Design review of the part built by this model. Coordinates are the model's own, in mm. Face numbers are marked on the shaded views. Round coordinates to 2 decimals unless told otherwise and drop trailing zeros. Order: outer loops, then holes, each group sorted by start corner. A loop starts at its lowest first (then second) coordinate and runs counter-clockwise, first axis right, second up.
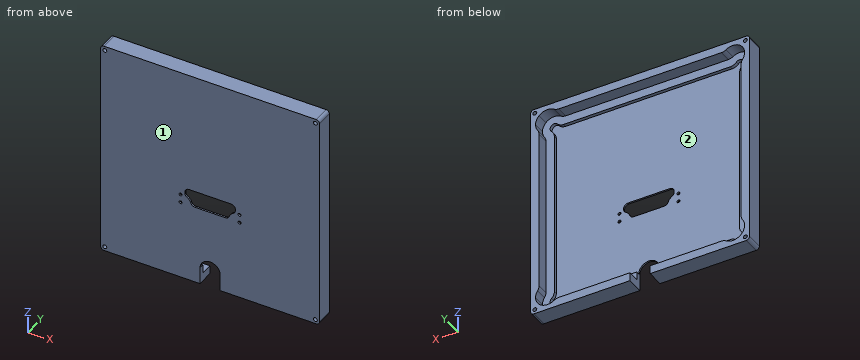
from build123d import *

# Parameters (mm, degrees)
SKETCH2_W           = 165.1
SKETCH2_H           = 165.1
BOSS_EXTRUDE1_DEPTH = 12.7
SKETCH3_W           = 152.4
SKETCH3_H           = 152.4
CUT_EXTRUDE1_DEPTH  = 8.9027
SKETCH4_W           = 139.7
SKETCH4_H           = 139.7
CUT_EXTRUDE2_DEPTH  = 2.54
SKETCH5_R           = 1.1303
CUT_EXTRUDE4_DEPTH  = 234.766882563
SKETCH6_R           = 1.4732
CUT_EXTRUDE5_DEPTH  = 234.831798522
FILLET2_R           = 2.54
CUT_EXTRUDE6_DEPTH  = 234.831798522
CUT_EXTRUDE11_DEPTH = 8.9027
SKETCH9_R           = 3.175
CUT_EXTRUDE12_DEPTH = 2.54
FILLET3_R           = 6.35
FILLET4_R           = 6.35
FILLET5_START       = -1
FILLET5_DEPTH       = 3
FILLET6_R           = 3.175


with BuildPart() as part:
    # Sketch2 → Boss-Extrude1 (new body)
    with BuildSketch(Plane(origin=(0, 0, 0), x_dir=(1, 0, 0), z_dir=(0, 1, 0))):
        with Locations((82.55, 82.55)):
            Rectangle(SKETCH2_W, SKETCH2_H)
    extrude(amount=BOSS_EXTRUDE1_DEPTH)

    # Sketch3 → Cut-Extrude1 (cut)
    with BuildSketch(Plane(origin=(0, 12.7, 0), x_dir=(1, 0, 0), z_dir=(0, 1, 0))):
        with Locations((82.55, 82.55)):
            Rectangle(SKETCH3_W, SKETCH3_H)
    extrude(amount=-CUT_EXTRUDE1_DEPTH, mode=Mode.SUBTRACT)

    # Sketch4 → Cut-Extrude2 (cut)
    with BuildSketch(Plane(origin=(0, 3.7973, 0), x_dir=(1, 0, 0), z_dir=(0, 1, 0))):
        with Locations((82.55, 82.55)):
            Rectangle(SKETCH4_W, SKETCH4_H)
    extrude(amount=-CUT_EXTRUDE2_DEPTH, mode=Mode.SUBTRACT)

    # Sketch5 → Cut-Extrude4 (cut, through all)
    with BuildSketch(Plane(origin=(0, 1.2573, 0), x_dir=(1, 0, 0), z_dir=(0, 1, 0))):
        with BuildLine():
            Line((93.98, 104.775), (71.12, 104.775))
            ThreePointArc((71.12, 104.775), (67.945, 101.6), (71.12, 98.425))
            Line((71.12, 98.425), (93.98, 98.425))
            ThreePointArc((93.98, 98.425), (97.155, 101.6), (93.98, 104.775))
        make_face()
        with Locations(Location((60.325, 98.425, 0), (0, 0, 270))):
            Circle(SKETCH5_R)
        with Locations(Location((104.775, 98.425, 0), (0, 0, 270))):
            Circle(SKETCH5_R)
        Polygon((101.6, 98.425), (93.98, 98.425), (71.12, 98.425), (63.5, 98.425), (63.5, 92.075), (101.6, 92.075), align=None)
        with Locations(Location((60.325, 104.775, 0), (0, 0, 270))):
            Circle(SKETCH5_R)
        with Locations(Location((104.775, 104.775, 0), (0, 0, 90))):
            Circle(SKETCH5_R)
    extrude(amount=-CUT_EXTRUDE4_DEPTH, mode=Mode.SUBTRACT)

    # Sketch6 → Cut-Extrude5 (cut, through all)
    with BuildSketch(Plane(origin=(0, 12.7, 0), x_dir=(1, 0, 0), z_dir=(0, 1, 0))):
        with Locations(Location((3.175, 161.925, 0), (0, 0, 270))):
            Circle(SKETCH6_R)
        with Locations(Location((161.925, 161.925, 0), (0, 0, 90))):
            Circle(SKETCH6_R)
        with Locations(Location((161.925, 3.175, 0), (0, 0, 270))):
            Circle(SKETCH6_R)
        with Locations(Location((3.175, 3.175, 0), (0, 0, 90))):
            Circle(SKETCH6_R)
    extrude(amount=-CUT_EXTRUDE5_DEPTH, mode=Mode.SUBTRACT)

    # Fillet2
    fillet2_edges = [part.edges().sort_by_distance(p)[0] for p in [
        (0, 6.35, -165.1),
        (165.1, 6.35, -165.1),
        (165.1, 6.35, 0),
        (0, 6.35, 0),
    ]]
    fillet(fillet2_edges, radius=FILLET2_R)

    # Sketch7 → Cut-Extrude6 (cut, through all)
    with BuildSketch(Plane(origin=(0, 12.7, 0), x_dir=(1, 0, 0), z_dir=(0, 1, 0))):
        with BuildLine():
            Line((74.93, 152.4), (74.93, 165.1))
            ThreePointArc((74.93, 165.1), (82.55, 172.72), (90.17, 165.1))
            Line((90.17, 165.1), (90.17, 152.4))
            ThreePointArc((90.17, 152.4), (82.55, 144.78), (74.93, 152.4))
        make_face()
    extrude(amount=-CUT_EXTRUDE6_DEPTH, mode=Mode.SUBTRACT)

    # Sketch8 → Cut-Extrude11 (cut)
    with BuildSketch(Plane(origin=(0, 12.7, 0), x_dir=(1, 0, 0), z_dir=(0, 1, 0))):
        with BuildLine():
            Line((6.35, 152.4), (6.35, 158.75))
            ThreePointArc((6.35, 158.75), (3.719743879, 152.4), (6.35, 146.05))
            Line((6.35, 146.05), (6.35, 152.4))
        make_face()
        with BuildLine():
            ThreePointArc((19.05, 158.75), (12.7, 161.380256121), (6.35, 158.75))
            Line((6.35, 158.75), (12.7, 158.75))
            Line((12.7, 158.75), (19.05, 158.75))
        make_face()
        with BuildLine():
            Line((6.35, 12.7), (6.35, 19.05))
            ThreePointArc((6.35, 19.05), (3.719743879, 12.7), (6.35, 6.35))
            Line((6.35, 6.35), (6.35, 12.7))
        make_face()
        with BuildLine():
            Line((12.7, 6.35), (6.35, 6.35))
            ThreePointArc((6.35, 6.35), (12.7, 3.719743879), (19.05, 6.35))
            Line((19.05, 6.35), (12.7, 6.35))
        make_face()
        with BuildLine():
            Line((152.4, 6.35), (146.05, 6.35))
            ThreePointArc((146.05, 6.35), (152.4, 3.719743879), (158.75, 6.35))
            Line((158.75, 6.35), (152.4, 6.35))
        make_face()
        with BuildLine():
            ThreePointArc((161.380256121, 12.7), (160.696674827, 16.136595236), (158.75, 19.05))
            Line((158.75, 19.05), (158.75, 12.7))
            Line((158.75, 12.7), (158.75, 6.35))
            ThreePointArc((158.75, 6.35), (160.696674827, 9.263404764), (161.380256121, 12.7))
        make_face()
        with BuildLine():
            Line((158.75, 152.4), (158.75, 146.05))
            ThreePointArc((158.75, 146.05), (160.696674827, 148.963404764), (161.380256121, 152.4))
            ThreePointArc((161.380256121, 152.4), (160.696674827, 155.836595236), (158.75, 158.75))
            Line((158.75, 158.75), (158.75, 152.4))
        make_face()
        with BuildLine():
            ThreePointArc((158.75, 158.75), (152.4, 161.380256121), (146.05, 158.75))
            Line((146.05, 158.75), (152.4, 158.75))
            Line((152.4, 158.75), (158.75, 158.75))
        make_face()
    extrude(amount=-CUT_EXTRUDE11_DEPTH, mode=Mode.SUBTRACT)

    # Sketch9 → Cut-Extrude12 (cut)
    with BuildSketch(Plane(origin=(0, 3.7973, 0), x_dir=(1, 0, 0), z_dir=(0, 1, 0))):
        with Locations((12.7, 152.4)):
            Circle(SKETCH9_R)
        with Locations((152.4, 152.4)):
            Circle(SKETCH9_R)
        with Locations((152.4, 12.7)):
            Circle(SKETCH9_R)
        with Locations((12.7, 12.7)):
            Circle(SKETCH9_R)
    extrude(amount=-CUT_EXTRUDE12_DEPTH, mode=Mode.SUBTRACT)

    # Fillet3
    fillet3_edges = [part.edges().sort_by_distance(p)[0] for p in [
        (149.225, 2.5273, -12.7),
        (15.875, 2.5273, -12.7),
        (152.4, 2.5273, -149.225),
        (12.7, 2.5273, -149.225),
        (12.7, 2.5273, -15.875),
        (152.4, 2.5273, -15.875),
        (149.225, 2.5273, -152.4),
        (15.875, 2.5273, -152.4),
    ]]
    fillet(fillet3_edges, radius=FILLET3_R)

    # Fillet4
    fillet4_edges = [part.edges().sort_by_distance(p)[0] for p in [
        (146.05, 8.24865, -158.75),
        (146.05, 8.24865, -6.35),
        (19.05, 8.24865, -6.35),
        (6.35, 8.24865, -146.05),
        (19.05, 8.24865, -158.75),
        (6.35, 8.24865, -19.05),
        (158.75, 8.24865, -19.05),
        (158.75, 8.24865, -146.05),
    ]]
    fillet(fillet4_edges, radius=FILLET4_R)

    # Fillet5: read off the stored shape, not the designer's step
    # Fillet5 outline → Fillet5 (cut)
    with BuildSketch(Plane(origin=(0, 0, 0), x_dir=(1, 0, 0), z_dir=(0, 1, 0)).offset(FILLET5_START)):
        with BuildLine():
            ThreePointArc((101.6, 98.425), (98.748828907, 99.911991034), (96.991709431, 102.605102634))
            ThreePointArc((96.991709431, 102.605102634), (96.556026578, 99.744006447), (93.98, 98.425))
            Line((93.98, 98.425), (101.6, 98.425))
        make_face()
        with BuildLine():
            ThreePointArc((68.108290569, 102.605102634), (66.351171093, 99.911991034), (63.5, 98.425))
            Line((63.5, 98.425), (71.12, 98.425))
            ThreePointArc((71.12, 98.425), (68.543973422, 99.744006447), (68.108290569, 102.605102634))
        make_face()
    extrude(amount=FILLET5_DEPTH, mode=Mode.SUBTRACT)

    # Fillet6
    fillet6_edges = [part.edges().sort_by_distance(p)[0] for p in [
        (101.6, 0.62865, -98.425),
        (101.6, 0.62865, -92.075),
        (63.5, 0.62865, -92.075),
        (63.5, 0.62865, -98.425),
    ]]
    fillet(fillet6_edges, radius=FILLET6_R)


solid = part.part
1) Clearance check with flat-ended pins moving along their axes: P1, Ø1, axis at x = 76, z = -62.5, coming from the +Y side; P2, Ø4.5, axis at x = 3.175, z = -161.925, coming from the +Y side; P3, Ø1.4, axis at x = 86, y = 0.5, coming from the -Z side. State where each tip first meets the part, or that it passes through.
Results:
P1: stops at y = 1.26
P2: stops at y = 12.7
P3: stops at z = -146.01
2) To check wall thickness, follow line 1 along X through (y, z) = (11.25, -32); line 2 along X through (y, z) = (2.25, -87); line 3 along Z through (x, y) = (94.5, 4.5). State the ranges of each line that lie inside material, in increasing order.
Results:
line 1: x = 0 to 6.35, 158.75 to 165.1
line 2: x = 0 to 12.7, 152.4 to 165.1
line 3: z = -165.1 to -158.75, -6.35 to 0
3) Take a section at D-D on y = 8.25. State how many separate pieces and enclosed holes the cut face has, plus the area to 3 significant figures.
Results:
separate pieces: 1
enclosed holes: 4
area: 3,710 mm2
4) Take a section at C-C on x = 45. Give the boundary of the cut face in (y, z), plus the area to 3 significant figures.
Results:
outline: (0, -165.1) - (12.7, -165.1) - (12.7, -158.75) - (3.8, -158.75) - (3.8, -152.4) - (1.26, -152.4) - (1.26, -12.7) - (3.8, -12.7) - (3.8, -6.35) - (12.7, -6.35) - (12.7, 0) - (0, 0) - close
area: 385 mm2
5) The part is to be moulded in two halves that separate along X. For the marked faces 1 and 2, say which applies: released by +X, released by -X, zero draft, split by the parting line, or undercut.
Results:
face 1: zero draft
face 2: undercut
6) Take a section at B-B on z = -78. Give the boundary of the cut face in (x, y).
Results:
outline: (0, 0) - (165.1, 0) - (165.1, 12.7) - (158.75, 12.7) - (158.75, 3.8) - (152.4, 3.8) - (152.4, 1.26) - (12.7, 1.26) - (12.7, 3.8) - (6.35, 3.8) - (6.35, 12.7) - (0, 12.7) - close
7) Take a section at A-A on x = 82.55. Give the boundary of the cut face in (y, z) (3 decimals).
Results:
outline: (0, -144.78) - (1.257, -144.78) - (1.257, -104.775) - (0, -104.775) - close; (0, -92.075) - (1.257, -92.075) - (1.257, -12.7) - (3.797, -12.7) - (3.797, -6.35) - (12.7, -6.35) - (12.7, 0) - (0, 0) - close
